The listing builds one solid part. Answer for the finished solid, in the listing's coordinates (mm). A direction names the side the tool comes from. Coordinates: 2 decimals unless noted, no trailing zeros. Write each loop counter-clockwise with the first axis right and the second up, starting at its lowest first coordinate (ties: lowest second). Pieces come first, ordered by that corner, then holes.
from build123d import *

# Parameters (mm, degrees)
F1_DEPTH = 62.45
F2_R     = 16.478049
F2_R_2   = 6
F3_DEPTH = 11.75
F4_R     = 15.413294
F4_R_2   = 6
F5_DEPTH = 11.75


with BuildPart() as f1:
    # F0 (on Front) → F1 (new body)
    with BuildSketch(Plane.XZ):
        Polygon((-4.907477, -8.5), (4.907477, -8.5), (9.814955, 0), (4.907477, 8.5), (-4.907477, 8.5), (-9.814955, 0), align=None)
    extrude(amount=-F1_DEPTH)

    # F2 (on face) → F3 (cut)
    with BuildSketch(Plane.XZ):
        Circle(F2_R)
        Circle(F2_R_2, mode=Mode.SUBTRACT)
    extrude(amount=-F3_DEPTH, mode=Mode.SUBTRACT)

    # F4 (on face) → F5 (cut)
    with BuildSketch(Plane(origin=(0, 62.45, 0), x_dir=(-1, 0, 0), z_dir=(0, 1, 0))):
        Circle(F4_R)
        Circle(F4_R_2, mode=Mode.SUBTRACT)
    extrude(amount=-F5_DEPTH, mode=Mode.SUBTRACT)


solid = f1.part
Q1. Given pin 1 (1 mm diameter, centred on y = 27, z = -3, fed in from +X); pin 2 (6 mm diameter, centred on y = 22, z = 6.5, fed in from -X); pin 3 (1 mm diameter, centred on y = 52, z = -3, fed in from -X), each flat-ended and moving along its own axis, determine where each tip first touches the part or whether it passes through.
Answers below:
pin 1: stops at x = 8.37
pin 2: stops at x = -7.79
pin 3: stops at x = -5.45
Q2. The part is cut by section C-C, the plane z = -2.5. Write down the section's boundary in (x, y).
Answers below:
outline: (-8.37, 11.75) - (-5.45, 11.75) - (-5.45, 0) - (5.45, 0) - (5.45, 11.75) - (8.37, 11.75) - (8.37, 50.7) - (5.45, 50.7) - (5.45, 62.45) - (-5.45, 62.45) - (-5.45, 50.7) - (-8.37, 50.7) - close
Q3. Which of the six approach directions +Z, -Z, +X, -X, +Y, -Y give full straight-line access (tool end or side, diameter ignored) to faces 1 (the face through (6, 57, 0)), 2 (the face through (0, 0, 0)), 3 (the face through (2, 11.75, 6))?
Answers below:
face 1: +Y
face 2: +Z, -Z, +X, -X, -Y
face 3: -Y
Q4. The part is cut by section A-A, the plane x = 0. Write down the section's boundary in (y, z), then the cut area to 3 significant figures.
Answers below:
outline: (0, -6) - (11.75, -6) - (11.75, -8.5) - (50.7, -8.5) - (50.7, -6) - (62.45, -6) - (62.45, 6) - (50.7, 6) - (50.7, 8.5) - (11.75, 8.5) - (11.75, 6) - (0, 6) - close
area: 944 mm2
Q5. Find the intervals of material crossed by probe 1 along Y at (x, z) = (-5.5, 6); probe 2 along X at (y, z) = (29.5, 6); probe 3 along Z at (x, y) = (2.75, 7.5), in increasing order.
Answers below:
probe 1: y = 11.75 to 50.7
probe 2: x = -6.35 to 6.35
probe 3: z = -5.33 to 5.33
Q6. The part is cut by section B-B, the plane y = 28. Write down the section's boundary in (x, z).
Answers below:
outline: (-9.81, 0) - (-4.91, -8.5) - (4.91, -8.5) - (9.81, 0) - (4.91, 8.5) - (-4.91, 8.5) - close
